```python
from build123d import *

# Parameters (mm, degrees)
SKETCH1_R           = 111.2139
SKETCH1_R_2         = 103.5939
BOSS_EXTRUDE1_DEPTH = 10.16
SKETCH2_R           = 111.2139
SKETCH2_R_2         = 43.815
BOSS_EXTRUDE3_DEPTH = 11.176
SKETCH3_R           = 48.895
SKETCH3_R_2         = 43.815
BOSS_EXTRUDE4_DEPTH = 50.8
FILLET1_R           = 2.54
FILLET2_R           = 2.54
SKETCH4_R           = 11.2776
CUT_EXTRUDE1_DEPTH  = 50.8
SKETCH5_R           = 6.6167
SKETCH5_R_2         = 4.0767
BOSS_EXTRUDE5_DEPTH = 10.16
FILLET3_R           = 2.54
SKETCH6_R           = 11.2776
SKETCH6_R_2         = 8.7376
BOSS_EXTRUDE6_DEPTH = 2.54


with BuildPart() as part:
    # Sketch1 → Boss-Extrude1 (new body)
    with BuildSketch(Plane.XY):
        Circle(SKETCH1_R)
        Circle(SKETCH1_R_2, mode=Mode.SUBTRACT)
    extrude(amount=BOSS_EXTRUDE1_DEPTH)

    # Sketch2 → Boss-Extrude3 (add)
    with BuildSketch(Plane(origin=(0, 0, 0), x_dir=(-1, 0, 0), z_dir=(0, 0, -1))):
        Circle(SKETCH2_R)
        Circle(SKETCH2_R_2, mode=Mode.SUBTRACT)
    extrude(amount=BOSS_EXTRUDE3_DEPTH)

    # Sketch3 → Boss-Extrude4 (add)
    with BuildSketch(Plane(origin=(0, 0, -11.176), x_dir=(-1, 0, 0), z_dir=(0, 0, -1))):
        Circle(SKETCH3_R)
        Circle(SKETCH3_R_2, mode=Mode.SUBTRACT)
    extrude(amount=BOSS_EXTRUDE4_DEPTH)

    # Fillet1
    fillet1_edges = [part.edges().sort_by_distance(p)[0] for p in [
        (-103.5939, 0, 0),
    ]]
    fillet(fillet1_edges, radius=FILLET1_R)

    # Fillet2
    fillet2_edges = [part.edges().sort_by_distance(p)[0] for p in [
        (48.895, 0, -11.176),
        (43.815, 0, 0),
        (111.2139, 0, -11.176),
    ]]
    fillet(fillet2_edges, radius=FILLET2_R)

    # Sketch4 → Cut-Extrude1 (cut)
    with BuildSketch(Plane(origin=(0, 0, -11.176), x_dir=(-1, 0, 0), z_dir=(0, 0, -1))):
        with Locations((0, -76.2)):
            Circle(SKETCH4_R)
    extrude(amount=-CUT_EXTRUDE1_DEPTH, mode=Mode.SUBTRACT)

    # Sketch5 → Boss-Extrude5 (add)
    with BuildSketch(Plane.XY):
        with Locations((0, 76.2)):
            Circle(SKETCH5_R)
        with Locations((0, 76.2)):
            Circle(SKETCH5_R_2, mode=Mode.SUBTRACT)
    extrude(amount=BOSS_EXTRUDE5_DEPTH)

    # Fillet3
    fillet3_edges = [part.edges().sort_by_distance(p)[0] for p in [
        (-6.6167, 76.2, 0),
    ]]
    fillet(fillet3_edges, radius=FILLET3_R)

    # Sketch6 → Boss-Extrude6 (add)
    with BuildSketch(Plane(origin=(0, 0, -11.176), x_dir=(-1, 0, 0), z_dir=(0, 0, -1))):
        with Locations((0, -76.2)):
            Circle(SKETCH6_R)
        with Locations((0, -76.2)):
            Circle(SKETCH6_R_2, mode=Mode.SUBTRACT)
    extrude(amount=-BOSS_EXTRUDE6_DEPTH)


solid = part.part
```
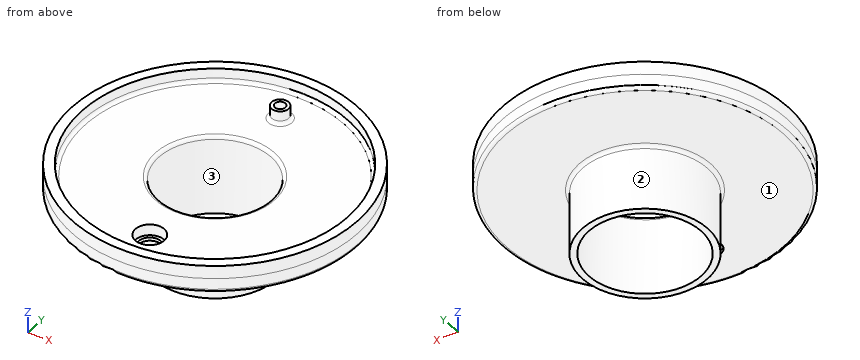
Can you work these out from the model? Positions are in its coordinate system, mm. Face numbers are marked on the shaded views. Coordinates: 2 decimals unless noted, no trailing zeros. Loops run counter-clockwise (first coordinate to the right, second up) from the corner with the lowest first, then second, coordinate; pieces in that order, holes last.
1) For pin 1 (25 mm diameter, centred on x = 5, y = -75.5, fed in from +Z); pin 2 (20 mm diameter, centred on x = 0, y = -76.2, fed in from -Z); pin 3 (12 mm diameter, centred on y = -18, z = -31, fed in from +X), each with a flat end and sliding along its axis, tell me the tip position at first contact or that it passes through.
2) Thinking about a two-plate mould opening in X: for the marked faces 1, 2 and 3, which applies, pulls with the +X half, pulls with the -X half, needs draft (parallel to the pull), parting line crosses it, or undercut?
3) I need wall thicknesses on probe 1 along Y at (x, z) = (0, 4.5); probe 2 along Y at (x, z) = (0, -6) (3 decimals); probe 3 along Y at (x, z) = (0, -39) (3 decimals). Which ranges of each line are inside material? Lowest first, please.
4) Imagine slicing it at B-B on x = 0. State how many separate pieces and enclosed holes the cut face has, plus the area to 3 significant figures.
5) Imagine slicing it at C-C on z = -49.5. List the corners of the cut face in (x, y) for me (3 decimals).
6) Imagine slicing it at A-A on y = 0. List the corners of the cut face in (x, z) for me (3 decimals), plus the area to 3 significant figures.
Completed:
1. pin 1: stops at z = 0
1. pin 2: stops at z = -11.18
1. pin 3: stops at x = 47.4
2. face 1: needs draft
2. face 2: parting line crosses it
2. face 3: undercut
3. probe 1: y = -111.21 to -103.59, 69.58 to 72.12, 80.28 to 82.82, 103.59 to 111.21
3. probe 2: y = -111.214 to -87.478, -64.922 to -43.815, 43.815 to 111.214
3. probe 3: y = -48.895 to -43.815, 43.815 to 48.895
4. separate pieces: 3
4. enclosed holes: 0
4. area: 1,990 mm2
5. outline: circle Ø97.79 at (0, 0); hole circle Ø87.63 at (0, 0)
6. outline: (-111.214, -8.636) arc R2.54 ccw to (-108.674, -11.176) - (-51.435, -11.176) arc R2.54 cw to (-48.895, -13.716) - (-48.895, -61.976) - (-43.815, -61.976) - (-43.815, -2.54) arc R2.54 ccw to (-46.355, 0) - (-101.054, 0) arc R2.54 cw to (-103.594, 2.54) - (-103.594, 10.16) - (-111.214, 10.16) - close; (43.815, -61.976) - (48.895, -61.976) - (48.895, -13.716) arc R2.54 cw to (51.435, -11.176) - (108.674, -11.176) arc R2.54 ccw to (111.214, -8.636) - (111.214, 10.16) - (103.594, 10.16) - (103.594, 2.54) arc R2.54 cw to (101.054, 0) - (46.355, 0) arc R2.54 ccw to (43.815, -2.54) - close
6. area: 2,180 mm2
